For this review, take the finished solid that the model builds, in its own axes (mm). Face numbers are marked on the shaded views. A direction names the side the tool comes from. Round coordinates to 2 decimals unless told otherwise and drop trailing zeros. Order: outer loops, then holes, each group sorted by start corner. A loop starts at its lowest first (then second) coordinate and runs counter-clockwise, first axis right, second up. Notation, with made-up numbers: M -7,19 L -1,19 A21 cw -1,49 Z; hole C 34,29 d1. An arc over 180 degrees is marked long. Answer as a JSON object with one key per item and string values.
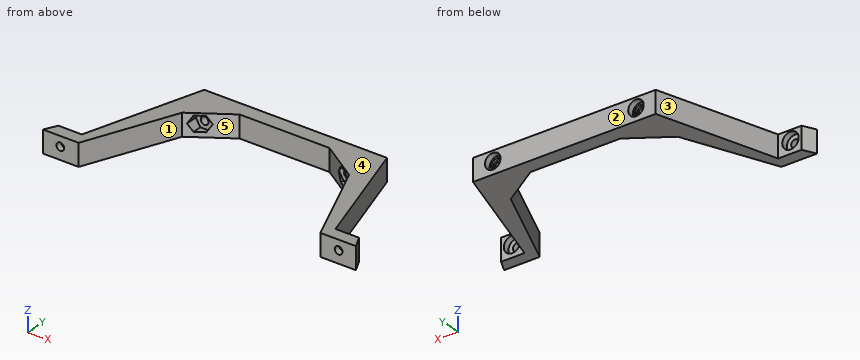
from build123d import *

# Parameters (mm, degrees)
EXTRUDE_1_DEPTH      = 10
SKETCH_7_R           = 1.55
CUT_EXTRUDE_1_DEPTH  = 49.544157215
CUT_EXTRUDE_2_DEPTH  = 8.5
SKETCH_19_W          = 126.714157214
SKETCH_19_H          = 0.99604336
CUT_EXTRUDE_14_DEPTH = 53.044157215
SKETCH_22_R          = 1.575
CUT_EXTRUDE_15_DEPTH = 10
SKETCH_23_R          = 3.35
CUT_EXTRUDE_16_DEPTH = 2.5


with BuildPart() as part:
    # 草图1 → 凸台-拉伸1 (new body)
    with BuildSketch(Plane.XY):
        Polygon((-3.188712924, 13.052848472), (33.811287076, 13.052848472), (33.811287076, 7.052848472), (15.60198174, 7.052848472), (0, -3.158579815), (-15.114428715, -38.991308743), (-29.545791531, -38.991308743), (-27.045791531, -33.991308743), (-17.548712924, -33.991308743), align=None)
    extrude_1 = extrude(amount=EXTRUDE_1_DEPTH)

    # 镜向1: 凸台-拉伸1 across plane
    add(extrude_1.mirror(Plane(origin=(33.811287076, 13.052848472, 10), x_dir=(0, 0, 1), z_dir=(-1, 0, 0))))

    # 草图5 → 切除-旋转7 (revolve, cut)
    with BuildSketch(Plane.XY.offset(5)):
        Polygon((7.961287076, 13.052848472), (7.961287076, 10.552848472), (7.161287076, 10.552848472), (7.161287076, 9.552848472), (6.361287076, 9.552848472), (4.811287076, 9.552848472), (4.811287076, 13.052848472), align=None)
    cut_revolve_7 = revolve(axis=Axis((4.811287076, 9.552848472, 5), (0, 1, 0)), mode=Mode.SUBTRACT)

    # 草图7 → 切除-拉伸1 (cut, through all)
    with BuildSketch(Plane(origin=(0, 9.552848472, 0), x_dir=(1, 0, 0), z_dir=(0, 1, 0))):
        with Locations((4.811287076, -5)):
            Circle(SKETCH_7_R)
    cut_extrude_1 = extrude(amount=-CUT_EXTRUDE_1_DEPTH, mode=Mode.SUBTRACT)

    # 草图8 → 切除-拉伸2 (cut)
    with BuildSketch(Plane(origin=(0, -5.947151528, 0), x_dir=(1, 0, 0), z_dir=(0, 1, 0))):
        Polygon((8.333123718, -5), (6.572205397, -1.95), (3.050368755, -1.95), (1.289450434, -5), (3.050368755, -8.05), (6.572205397, -8.05), align=None)
    cut_extrude_2 = extrude(amount=CUT_EXTRUDE_2_DEPTH, mode=Mode.SUBTRACT)

    # 草图19 → 切除-拉伸14 (cut, through all)
    with BuildSketch(Plane(origin=(0, 13.052848472, 0), x_dir=(1, 0, 0), z_dir=(0, 1, 0))):
        with Locations((33.811287076, -9.50197832)):
            Rectangle(SKETCH_19_W, SKETCH_19_H)
    extrude(amount=-CUT_EXTRUDE_14_DEPTH, mode=Mode.SUBTRACT)

    # 草图22 → 切除-拉伸15 (cut)
    with BuildSketch(Plane(origin=(0, -33.991308743, 0), x_dir=(1, 0, 0), z_dir=(0, 1, 0))):
        with Locations((-22.548712924, -5.00395664)):
            Circle(SKETCH_22_R)
    cut_extrude_15 = extrude(amount=-CUT_EXTRUDE_15_DEPTH, mode=Mode.SUBTRACT)

    # 草图23 → 切除-拉伸16 (cut)
    with BuildSketch(Plane(origin=(0, -33.991308743, 0), x_dir=(1, 0, 0), z_dir=(0, 1, 0))):
        with Locations((-22.548712924, -5.00395664)):
            Circle(SKETCH_23_R)
    cut_extrude_16 = extrude(amount=-CUT_EXTRUDE_16_DEPTH, mode=Mode.SUBTRACT)

    # 镜向2: 切除-旋转7, 切除-拉伸1, 切除-拉伸2, 切除-拉伸15, 切除-拉伸16 across plane
    add(cut_revolve_7.mirror(Plane(origin=(33.811287076, 0, 0), x_dir=(0, 0, 1), z_dir=(1, 0, 0))), mode=Mode.SUBTRACT)
    add(cut_extrude_1.mirror(Plane(origin=(33.811287076, 0, 0), x_dir=(0, 0, 1), z_dir=(1, 0, 0))), mode=Mode.SUBTRACT)
    add(cut_extrude_2.mirror(Plane(origin=(33.811287076, 0, 0), x_dir=(0, 0, 1), z_dir=(1, 0, 0))), mode=Mode.SUBTRACT)
    add(cut_extrude_15.mirror(Plane(origin=(33.811287076, 0, 0), x_dir=(0, 0, 1), z_dir=(1, 0, 0))), mode=Mode.SUBTRACT)
    add(cut_extrude_16.mirror(Plane(origin=(33.811287076, 0, 0), x_dir=(0, 0, 1), z_dir=(1, 0, 0))), mode=Mode.SUBTRACT)


solid = part.part
1) Mouldability with a two-part tool opening along X and no side actions: class the marked faces 3, 4 and 5 as +X half, -X half, draft (parallel to the pull), parting line (faces both ways), or undercut.
Geometry check:
{"face 3": "-X half", "face 4": "draft", "face 5": "undercut"}
2) Add section C-C on x = 79.5. State the section outline as (y, z) points, and give its area (3 significant figures).
Geometry check:
{"outline": "M -31.32,0 L -15.41,0 L -15.41,9 L -31.32,9 Z", "area": "143 mm²"}
3) Add section A-A on y = -11. State the section outline as (x, z) points, and give its area (3 significant figures).
Geometry check:
{"outline": "M -10.53,0 L -3.31,0 L -3.31,9 L -10.53,9 Z; M 70.93,0 L 78.15,0 L 78.15,9 L 70.93,9 Z", "area": "130 mm²"}
4) Machinability: for the marked faces 1 and 2, which of the approach directions +Z, -Z, +X, -X, +Y, -Y give a long, thin tool a straight path to every point of the face, cutting with its end or side? Answer none if there is none.
Geometry check:
{"face 1": "+Z, -Z, -Y", "face 2": "+Z, -Z, +X, -X, +Y"}
5) For L1, parallel to X at y = 11.8, z = 5; L2, parallel to Y at x = 3, z = 7.5; L3, parallel to X at y = -29, z = 1.5, list the stretches that pass through material, from the lowest coordinate up.
Geometry check:
{"L1": "x = -3.57 to 1.66, 7.96 to 59.66, 65.96 to 71.19", "L2": "y = 2.55 to 10.55", "L3": "x = -16.03 to -10.9, 78.52 to 83.65"}
6) Add section B-B on y = -18.5. State the section outline as (x, z) points.
Geometry check:
{"outline": "M -12.82,0 L -6.47,0 L -6.47,9 L -12.82,9 Z; M 74.09,0 L 80.44,0 L 80.44,9 L 74.09,9 Z"}
7) Insertion check: P1, Ø2.5, axis at x = 62.5, z = 4, coming from the +Y side; P2, Ø1, axis at y = -27, z = 3, coming from the -X side; P3, Ø3.5, axis at x = -22.55, z = 5, coming from the +Y side; P4, Ø3, axis at x = 5.5, y = 1, coming from the -Z side. Each pin has a flat end and moves straight along its axis. Give the tip position at first contact, or say it passes through.
Geometry check:
{"P1": "stops at y = 9.55", "P2": "stops at x = -15.57", "P3": "stops at y = -36.49", "P4": "stops at z = 0"}
